Here's how the part is built. I have some questions about the finished solid (model axes, mm). Face numbers are marked on the shaded views. A direction names the side the tool comes from. Round coordinates to 2 decimals unless told otherwise and drop trailing zeros. Order: outer loops, then holes, each group sorted by start corner. A loop starts at its lowest first (then second) coordinate and runs counter-clockwise, first axis right, second up. Notation, with made-up numbers: (38.25, 68) - (56.25, 68) arc R17 cw to (56.25, 81) - close; hole circle Ø11 at (52, 77). An arc over 180 degrees is marked (long way). Answer as a JSON object with one key per item and string values.
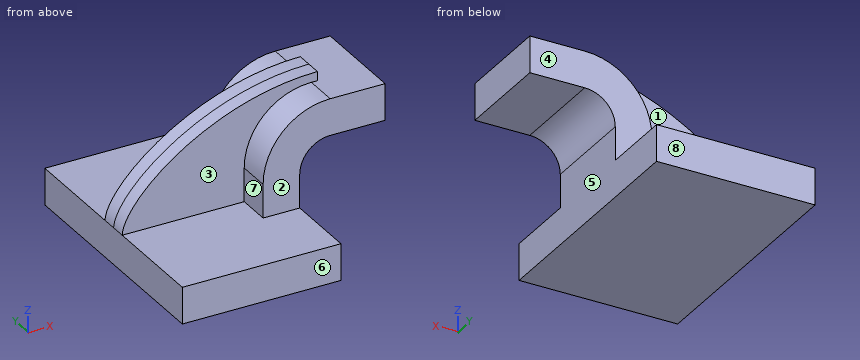
```python
from build123d import *

# Parameters (mm, degrees)
F1_DEPTH = 63.5
F0_W     = 25.4
F0_H     = 19.05
F2_DEPTH = 25.4
F3_DEPTH = 7.9375


# Not quite as in the source:
# - a feature of the source that left no trace in its solid (it failed there, or was rolled back) is left out


with BuildPart() as f1:
    # F0 (on Front) → F1 (new body, symmetric)
    with BuildSketch(Plane.XZ):
        Polygon((-41.275, -9.525), (41.275, -9.525), (41.275, 9.525), (22.225, 9.525), (-41.275, 9.525), align=None)
    extrude(amount=F1_DEPTH, both=True)

    # F0 (on Front) → F2 (join, symmetric)
    with BuildSketch(Plane.XZ):
        with BuildLine():
            Line((22.225, 9.525), (41.275, 9.525))
            Line((41.275, 9.525), (41.275, 27.0002))
            ThreePointArc((41.275, 27.0002), (45.9246798487, 38.2255201513), (57.15, 42.8752))
            Line((57.15, 42.8752), (60.325, 42.8752))
            Line((60.325, 42.8752), (60.325, 61.9252))
            Line((60.325, 61.9252), (57.15, 61.9252))
            ThreePointArc((57.15, 61.9252), (32.4542956671, 51.6959043329), (22.225, 27.0002))
            Line((22.225, 27.0002), (22.225, 9.525))
        make_face()
        with Locations((73.025, 52.4002)):
            Rectangle(F0_W, F0_H)
    extrude(amount=F2_DEPTH, both=True)

    # F0 (on Front) → F3 (join, symmetric)
    with BuildSketch(Plane.XZ):
        with BuildLine():
            add(Edge.make_bspline(
                [(-41.275, 9.525), (-40.3944440186, 27.1777566522), (4.0625981055, 66.2999525666), (60.325, 66.675)],
                knots=[0, 0, 0, 0, 116.5705044169, 116.5705044169, 116.5705044169, 116.5705044169], degree=3))
            Line((-41.275, 9.525), (22.225, 9.525))
            Line((22.225, 9.525), (22.225, 27.0002))
            ThreePointArc((22.225, 27.0002), (32.4542956671, 51.6959043329), (57.15, 61.9252))
            Line((57.15, 61.9252), (60.325, 61.9252))
            Line((60.325, 61.9252), (60.325, 66.675))
        make_face()
    extrude(amount=F3_DEPTH, both=True)


solid = f1.part
```
1. For P1, Ø14.5, axis at x = 70.5, y = 11, coming from the -Z side; P2, Ø5, axis at y = -16, z = 15.5, coming from the -X side (3 decimals); P3, Ø2, axis at y = -3.5, z = 42.5, coming from the +X side (3 decimals); P4, Ø3, axis at x = 39.5, y = -49, coming from the +Z side (3 decimals), each with a flat end and sliding along its axis, tell me the tip position at first contact or that it passes through.
Responses:
{"P1": "z = 42.88", "P2": "x = 22.225", "P3": "x = 85.725", "P4": "z = 9.525"}
2. Imagine slicing it at B-B (z = 4.5). List the corners of the cut face in (x, y) for me (3 decimals).
Responses:
{"outline": "(-41.275, -63.5) - (41.275, -63.5) - (41.275, 63.5) - (-41.275, 63.5) - close"}
3. If I drill on L1, parallel to Y at x = 14, z = 23; L2, parallel to Z at x = -16.5, y = 23.5 (3 decimals); L3, parallel to Y at x = 27.5, z = 21, over which ranges is the centre line in solid material (lowest first)? Write a range as [from, to].
Responses:
{"L1": "[-7.94, 7.94]", "L2": "[-9.525, 9.525]", "L3": "[-25.4, 25.4]"}
4. For the marked faces 1, 2, 3, 4 and 5, which set-ups out of +Z, -Z, +X, -X, +Y, -Y let a thin tool reach every point of the face, with its end or its side?
Responses:
{"face 1": "+Z, -X, +Y", "face 2": "+Z, +X, -X, -Y", "face 3": "+Z, -X, -Y", "face 4": "+Z, +X, -X, +Y", "face 5": "-Z, +X, +Y, -Y"}
5. Imagine slicing it at C-C (y = 44). List the corners of the cut face in (x, z) for me (3 decimals), plus the area to 3 significant figures.
Responses:
{"outline": "(-41.275, -9.525) - (41.275, -9.525) - (41.275, 9.525) - (-41.275, 9.525) - close", "area": "1,570 mm2"}
6. Imagine slicing it at A-A (y = 13). List the corners of the cut face in (x, z) for me (3 decimals).
Responses:
{"outline": "(-41.275, -9.525) - (41.275, -9.525) - (41.275, 27) arc R15.875 cw to (57.15, 42.875) - (85.725, 42.875) - (85.725, 61.925) - (57.15, 61.925) arc R34.925 ccw to (22.225, 27) - (22.225, 9.525) - (-41.275, 9.525) - close"}
7. Thinking about a two-plate mould opening in Y: for the marked faces 6, 7 and 8, which applies, pulls with the +Y half, pulls with the -Y half, needs draft (parallel to the pull), parting line crosses it, or undercut?
Responses:
{"face 6": "pulls with the -Y half", "face 7": "needs draft", "face 8": "pulls with the +Y half"}
